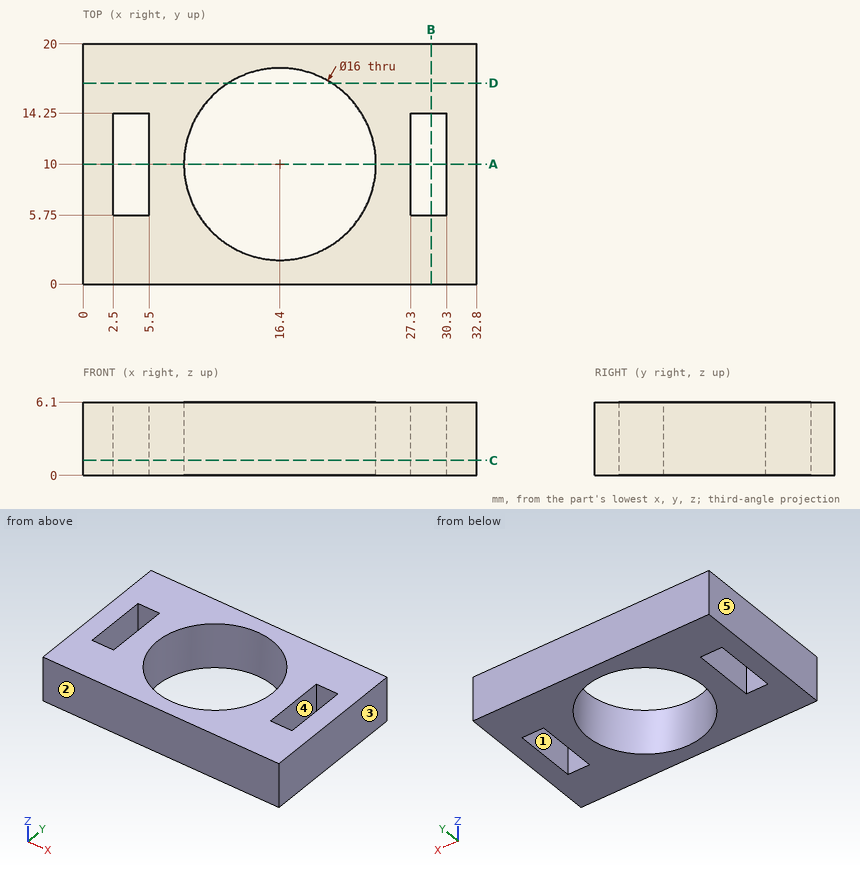
For this review, use the dimensioned drawing (mm, ordinates from the lowest corner) and the shaded views. A direction names the side the tool comes from. Give positions to 0.01 mm unless a question says otherwise; leave off trailing zeros. Order: outer loops, then holes, each group sorted by start corner. A loop starts at its lowest first (then second) coordinate and runs counter-clockwise, first axis right, second up. Notation, with made-up numbers: M -12,48 L 45,48 A19 cw 45,52 Z; hole C -9,84 d4. An arc over 180 degrees is marked long. Use one line per item in the form item = value. Start each with the question number.
Item 1: The part is to be moulded in two halves that separate along X. For the marked faces 1, 2 and 3, say which applies: pulls with the +X half, pulls with the -X half, needs draft (parallel to the pull), parting line crosses it, or undercut.
Item 2: We need section A-A on y = 10. Give the boundary of the cut face in (x, z).
Item 3: To check wall thickness, follow line 1 along Y through (x, z) = (16.4, 2.5); line 2 along X through (y, z) = (7.5, 3.25); line 3 along X through (y, z) = (13, 2.25). State the ranges of each line that lie inside material, in increasing order. Write a range as from..to.
Item 4: Insertion check: pin 1 Ø4 at (x, y) = (12, 14) entering from +Z. The pin has a flat end and moves straight along its axis. Give the tip position at first contact, or say it passes through.
Item 5: For the marked faces 4 and 5, list the 3-axis set-ups (+Z, -Z, +X, -X, +Y, -Y) from which the entire face can be reached by the end or side of a thin tool; tool diameter is ignored.
Item 6: We need section C-C on z = 1.25. Give the boundary of the cut face in (x, y), plus the area to 3 significant figures.
Item 7: We need section B-B on x = 29. Give the boundary of the cut face in (y, z).
Item 8: We need section D-D on y = 16.75. Give the boundary of the cut face in (x, z).
Completed:
q1.face_1 = undercut
q1.face_2 = needs draft
q1.face_3 = pulls with the +X half
q2.outline = M 0,0 L 2.5,0 L 2.5,6.1 L 0,6.1 Z; M 5.5,0 L 8.4,0 L 8.4,6.1 L 5.5,6.1 Z; M 24.4,0 L 27.3,0 L 27.3,6.1 L 24.4,6.1 Z; M 30.3,0 L 32.8,0 L 32.8,6.1 L 30.3,6.1 Z
q3.line_1 = 0..2, 18..20
q3.line_2 = 0..2.5, 5.5..8.8, 24..27.3, 30.3..32.8
q3.line_3 = 0..2.5, 5.5..8.98, 23.82..27.3, 30.3..32.8
q4.pin_1 = through
q5.face_4 = +Z, -Z
q5.face_5 = +Z, -Z, -X, +Y, -Y
q6.outline = M 0,0 L 32.8,0 L 32.8,20 L 0,20 Z; hole M 2.5,5.75 L 5.5,5.75 L 5.5,14.25 L 2.5,14.25 Z; hole C 16.4,10 d16; hole M 27.3,5.75 L 30.3,5.75 L 30.3,14.25 L 27.3,14.25 Z
q6.area = 404 mm²
q7.outline = M 0,0 L 5.75,0 L 5.75,6.1 L 0,6.1 Z; M 14.25,0 L 20,0 L 20,6.1 L 14.25,6.1 Z
q8.outline = M 0,0 L 12.11,0 L 12.11,6.1 L 0,6.1 Z; M 20.69,0 L 32.8,0 L 32.8,6.1 L 20.69,6.1 Z
